```python
from build123d import *

# Parameters (mm, degrees)
SKETCH1_R           = 1.6
BOSS_EXTRUDE1_DEPTH = 20
SKETCH2_W           = 15
SKETCH2_H           = 7
CUT_EXTRUDE1_DEPTH  = 34.541019662


with BuildPart() as part:
    # Sketch1 → Boss-Extrude1 (new body)
    with BuildSketch(Plane.XY):
        with BuildLine():
            Line((-20, 5), (0, 5))
            ThreePointArc((0, 5), (5, 0), (0, -5))
            Line((0, -5), (-20, -5))
            ThreePointArc((-20, -5), (-25, 0), (-20, 5))
        make_face()
        with Locations((-20, 0)):
            Circle(SKETCH1_R, mode=Mode.SUBTRACT)
        Circle(SKETCH1_R, mode=Mode.SUBTRACT)
    extrude(amount=BOSS_EXTRUDE1_DEPTH)

    # Sketch2 → Cut-Extrude1 (cut, through all)
    with BuildSketch(Plane(origin=(0, 5, 0), x_dir=(1, 0, 0), z_dir=(0, 1, 0))):
        with Locations((-17.5, -6.5)):
            Rectangle(SKETCH2_W, SKETCH2_H)
    extrude(amount=-CUT_EXTRUDE1_DEPTH, mode=Mode.SUBTRACT)


solid = part.part
```
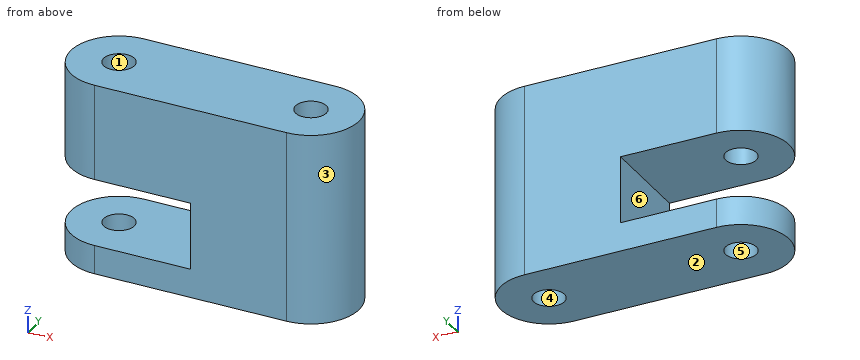
Here's how the part is built. I have some questions about the finished solid (model axes, mm). Face numbers are marked on the shaded views. A direction names the side the tool comes from. Coordinates: 2 decimals unless noted, no trailing zeros. Order: outer loops, then holes, each group sorted by start corner. A loop starts at its lowest first (then second) coordinate and runs counter-clockwise, first axis right, second up.
Item 1: Thinking about a two-plate mould opening in X: for the marked faces 1, 2, 3 and 4, which applies, pulls with the +X half, pulls with the -X half, needs draft (parallel to the pull), parting line crosses it, or undercut?
Response values:
face 1: undercut
face 2: needs draft
face 3: pulls with the +X half
face 4: undercut
Item 2: Which directions (+Z, -Z, +X, -X, +Y, -Y) give clear straight access to the entire face, cutting with the end or side of a thin tool? Please do the marked faces 5 and 6.
Response values:
face 5: +Z, -Z
face 6: -X, +Y, -Y
Item 3: If we section it at B-B, the plane y = -0.5: List the corners of the cut face in (x, z) for me.
Response values:
outline: (-24.97, 0) - (-21.52, 0) - (-21.52, 3) - (-24.97, 3) - close; (-24.97, 10) - (-21.52, 10) - (-21.52, 20) - (-24.97, 20) - close; (-18.48, 0) - (-1.52, 0) - (-1.52, 20) - (-18.48, 20) - (-18.48, 10) - (-10, 10) - (-10, 3) - (-18.48, 3) - close; (1.52, 0) - (4.97, 0) - (4.97, 20) - (1.52, 20) - close
Item 4: If we section it at D-D, the plane z = 18.5: List the corners of the cut face in (x, y) for me.
Response values:
outline: (-20, -5) - (0, -5) arc R5 ccw to (0, 5) - (-20, 5) arc R5 ccw to start; hole circle Ø3.2 at (-20, 0); hole circle Ø3.2 at (0, 0)
Item 5: I need wall thicknesses on probe 1 along Y at (x, z) = (-20, 0.95); probe 2 along Z at (x, y) = (-23, -3.75); probe 3 along X at (y, z) = (1.25, 18). Which ranges of each line are inside material? Lowest first, please.
Response values:
probe 1: y = -5 to -1.6, 1.6 to 5
probe 2: z = 0 to 3, 10 to 20
probe 3: x = -24.84 to -21, -19 to -1, 1 to 4.84
Item 6: If we section it at A-A, the plane x = -16.5: List the corners of the cut face in (y, z) for me.
Response values:
outline: (-5, 0) - (5, 0) - (5, 3) - (-5, 3) - close; (-5, 10) - (5, 10) - (5, 20) - (-5, 20) - close
Item 7: I'm going to push flat-ended pins straight in: pin 1 Ø1 at (y, z) = (1, 4) entering from +X; pin 2 Ø3.5 at (y, z) = (1.5, 6) entering from -X. Where does each tip first touch, or does it pass through?
Response values:
pin 1: stops at x = 4.97
pin 2: stops at x = -10
Item 8: If we section it at C-C, the plane z = 6: List the corners of the cut face in (x, y) for me, then the cut area to 3 significant figures.
Response values:
outline: (-10, -5) - (0, -5) arc R5 ccw to (0, 5) - (-10, 5) - close; hole circle Ø3.2 at (0, 0)
area: 131 mm2
